Autodesk Fusion 360 part; units mm, degrees
sketch "Sketch1" plane through (0, 0, 0) normal (0, 0, 1) x (1, 0, 0)
  line L0 (2, 0) -> (126.5, 0)
  line L1 (128.5, 2) -> (128.5, 75)
  line L2 (126.5, 77) -> (2, 77)
  line L3 (0, 75) -> (0, 2)
  line L4 (0, 74.5) -> (128.5, 74.5) construction
  line L5 (0, 2.5) -> (128.5, 2.5) construction
  line L6 (126, 77) -> (126, 0) construction
  line L7 (2.5, 77) -> (2.5, 0) construction
  circle A0 centre (2.5, 74.5) radius 1.5
  circle A1 centre (126, 74.5) radius 1.5
  circle A2 centre (126, 2.5) radius 1.5
  circle A3 centre (2.5, 2.5) radius 1.5
  arc A4 (2, 77) -> (0, 75) centre (2, 75) ccw
  arc A5 (128.5, 75) -> (126.5, 77) centre (126.5, 75) ccw
  arc A6 (126.5, 0) -> (128.5, 2) centre (126.5, 2) ccw
  arc A7 (0, 2) -> (2, 0) centre (2, 2) ccw
  point P0 (128.5, 0)
  point P1 (0, 77)
  dimension "d1" = 128.5
  dimension "d2" = 77
  dimension "d4" = 3
  dimension "d5" = 3
  dimension "d6" = 3
  dimension "d7" = 3
  dimension "d8" = 2.5
  dimension "d9" = 2.5
  dimension "d10" = 2.5
  dimension "d11" = 2.5
  dimension "d12" = 2
  dimension "d13" = 2
  dimension "d14" = 2
  dimension "d15" = 2
extrude "Extrude1" add sketch "Sketch1" along normal blind 1.5
sketch "Sketch2" plane through (0, 0, 1.5) normal (0, 0, 1) x (-1, 0, 0)
  circle A0 centre (-2.5, -74.5) radius 1.5
  circle A1 centre (-2.5, -2.5) radius 1.5
  circle A2 centre (-126, -2.5) radius 1.5
  circle A3 centre (-126, -74.5) radius 1.5
  arc A4 (0, -2) -> (-2, 0) centre (-2, -2) ccw
  line L0 (-2, 0) -> (-126.5, 0)
  arc A5 (-126.5, 0) -> (-128.5, -2) centre (-126.5, -2) ccw
  line L1 (-128.5, -2) -> (-128.5, -75)
  arc A6 (-128.5, -75) -> (-126.5, -77) centre (-126.5, -75) ccw
  line L2 (-126.5, -77) -> (-2, -77)
  arc A7 (-2, -77) -> (0, -75) centre (-2, -75) ccw
  line L3 (0, -75) -> (0, -2)
  line L4 (0, -38.5) -> (-128.5, -38.5) construction
  line L5 (-64.25, -77) -> (-64.25, 0) construction
  line L6 (-58.75, -22.5) -> (-69.75, -22.5)
  line L7 (-69.75, -22.5) -> (-69.75, -54.5)
  line L8 (-69.75, -54.5) -> (-58.75, -54.5)
  line L9 (-58.75, -54.5) -> (-58.75, -22.5)
  line L10 (-58.75, -22.5) -> (-69.75, -54.5) construction
  line L11 (-69.75, -22.5) -> (-58.75, -54.5) construction
  point P0 (-64.25, -38.5)
  dimension "d18" = 11
  dimension "d19" = 32
extrude "Extrude2" add sketch "Sketch2" along normal blind 13 contours L6 L7 L8 L9
sketch "Sketch3" plane through (58.75, 0, 0) normal (-1, 0, 0) x (0, -1, 0)
  line L0 (-54.5, 1.5) -> (-22.5, 1.5)
  line L1 (-22.5, 1.5) -> (-22.5, 14.5)
  line L2 (-22.5, 14.5) -> (-54.5, 14.5)
  line L3 (-54.5, 14.5) -> (-54.5, 1.5)
  line L4 (-54.5, 8) -> (-22.5, 8) construction
  line L5 (-38.5, 14.5) -> (-38.5, 1.5) construction
  line L6 (-24.25, 3) -> (-52.75, 3)
  line L7 (-52.75, 3) -> (-52.75, 13)
  line L8 (-52.75, 13) -> (-24.25, 13)
  line L9 (-24.25, 13) -> (-24.25, 3)
  line L10 (-24.25, 3) -> (-52.75, 13) construction
  line L11 (-52.75, 3) -> (-24.25, 13) construction
  line L12 (-25.25, 11.75) -> (-51.75, 11.75)
  line L13 (-51.75, 11.75) -> (-51.75, 4.25)
  line L14 (-51.75, 4.25) -> (-25.25, 4.25)
  line L15 (-25.25, 4.25) -> (-25.25, 11.75)
  line L16 (-25.25, 11.75) -> (-51.75, 4.25) construction
  line L17 (-51.75, 11.75) -> (-25.25, 4.25) construction
  point P0 (-38.5, 8)
  point P1 (-38.5, 8)
  dimension "d22" = 28.5
  dimension "d23" = 10
  dimension "d24" = 26.5
  dimension "d25" = 7.5
extrude "Extrude3" cut sketch "Sketch3" against normal blind 30 contours L12 L13 L14 L15
extrude "Extrude4" cut sketch "Sketch3" against normal blind 9.5 contours L6 L7 L8 L9
fillet "Fillet1" radius 2 1 edges at (64.25, 22.5, 1.5)
fillet "Fillet2" radius 2 1 edges at (64.25, 54.5, 1.5)
equation "mounting_hole = 3 mm"
equation "d4 = mounting_hole"
equation "d5 = mounting_hole"
equation "d6 = mounting_hole"
equation "d7 = mounting_hole"
Could you check a few things on this model? Use its own coordinates, in mm. A direction names the side the tool comes from. Round coordinates to 2 decimals unless told otherwise and drop trailing zeros. Order: outer loops, then holes, each group sorted by start corner. A loop starts at its lowest first (then second) coordinate and runs counter-clockwise, first axis right, second up.
(1) Imagine slicing it at D-D (x = 110). Write out the boundary of the cut face in (y, z).
Response values:
outline: (0, 0) - (77, 0) - (77, 1.5) - (0, 1.5) - close
(2) Imagine slicing it at C-C (y = 11). Write out the boundary of the cut face in (x, z), plus the area to 3 significant figures.
Response values:
outline: (0, 0) - (128.5, 0) - (128.5, 1.5) - (0, 1.5) - close
area: 193 mm2
(3) Which directions (+Z, -Z, +X, -X, +Y, -Y) give clear straight access to the entire face, cutting with the end or side of a thin tool? Please do faces 1 (the flat face through (58.75, 37.3, 13.3)), 2 (the flat face through (64, 22.5, 9)), 3 (the flat face through (69.75, 42, 4)), 4 (the flat face through (64, 54.5, 9)), 5 (the flat face through (63, 38, 3)).
Response values:
face 1: +Z, -X, +Y, -Y
face 2: +Z, +X, -X, -Y
face 3: +Z, +X, +Y, -Y
face 4: +Z, +X, -X, +Y
face 5: -X
(4) Imagine slicing it at B-B (y = 43). Write out the boundary of the cut face in (x, z).
Response values:
outline: (0, 0) - (128.5, 0) - (128.5, 1.5) - (69.75, 1.5) - (69.75, 4.25) - (68.25, 4.25) - (68.25, 3) - (58.75, 3) - (58.75, 1.5) - (0, 1.5) - close; (58.75, 13) - (68.25, 13) - (68.25, 11.75) - (69.75, 11.75) - (69.75, 14.5) - (58.75, 14.5) - close
(5) If we mould it in two halves opening along Z, with no side actions, what happens to faces 6 (the flat face through (63, 39, 13)), 7 (the cylindrical face through (124.5, 74.43, 0.74)), 8 (the flat face through (63, 52.75, 8)), 9 (the flat face through (78, 39, 1.5))? For each: released by +Z, released by -Z, zero draft, split by the parting line, or undercut.
Response values:
face 6: undercut
face 7: zero draft
face 8: undercut
face 9: released by +Z
(6) Please list where these lines run through material, in increasing order: line 1 along Y through (x, z) = (2.5, 0.5); line 2 along X through (y, z) = (74.5, 0.3); line 3 along Z through (x, y) = (95, 17).
Response values:
line 1: y = 0 to 1, 4 to 73, 76 to 77
line 2: x = 0 to 1, 4 to 124.5, 127.5 to 128.5
line 3: z = 0 to 1.5
(7) I'm going to push flat-ended pins straight in: pin 1 (1.6 mm diameter, centred on x = 69, z = 8.5, fed in from -Y); pin 2 (5 mm diameter, centred on x = 97, y = 10, fed in from +Z); pin 3 (6.5 mm diameter, centred on y = 41, z = 11, fed in from +X). Where does each tip first touch, or does it pass through?
Response values:
pin 1: stops at y = 22.5
pin 2: stops at z = 1.5
pin 3: stops at x = 69.75
(8) Imagine slicing it at A-A (z = 6.25). Write out the boundary of the cut face in (x, y).
Response values:
outline: (58.75, 22.5) - (69.75, 22.5) - (69.75, 25.25) - (68.25, 25.25) - (68.25, 24.25) - (58.75, 24.25) - close; (58.75, 52.75) - (68.25, 52.75) - (68.25, 51.75) - (69.75, 51.75) - (69.75, 54.5) - (58.75, 54.5) - close
